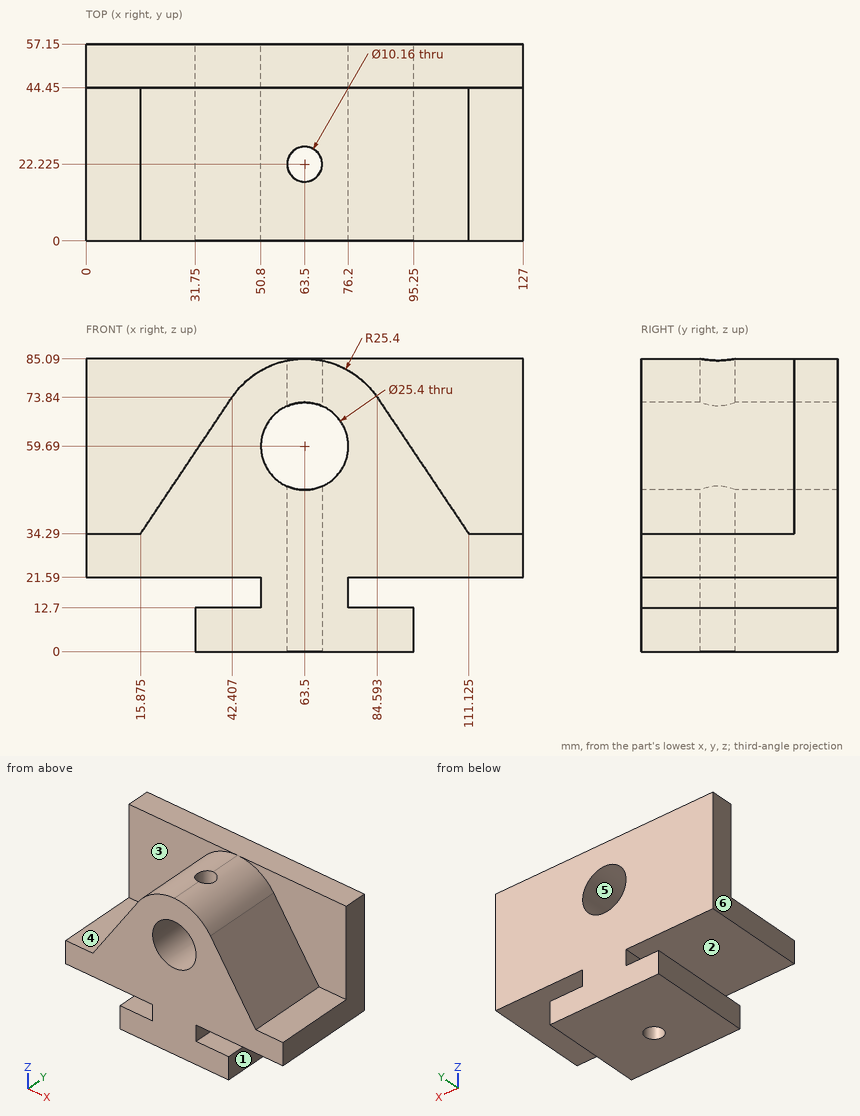
For this review, use the dimensioned drawing (mm, ordinates from the lowest corner) and the shaded views. A direction names the side the tool comes from. Give positions to 0.01 mm unless a question says otherwise; leave off trailing zeros. Use one line per item in the form item = value. Start each with the question number.
Item 1: To check wall thickness, follow line 1 along Z through (x, y) = (90.5, 46.5); line 2 along Z through (x, y) = (63.5, 12); line 3 along Y through (x, z) = (63, 76). State the ranges of each line that lie inside material, in increasing order. Write a range as from..to.
Item 2: For the marked faces 1, 2 and 3, list the 3-axis set-ups (+Z, -Z, +X, -X, +Y, -Y) from which the entire face can be reached by the end or side of a thin tool; tool diameter is ignored.
Item 3: Insertion check: pin 1 Ø1.5 at (x, y) = (36, 19.5) entering from +Z; pin 2 Ø5 at (x, y) = (25, 33) entering from +Z; pin 3 Ø15 at (x, y) = (86, 24) entering from +Z. Each pin has a flat end and moves straight along its axis. Give the tip position at first contact, or say it passes through.
Item 4: The part is to be moulded in two halves that separate along X. For the marked faces 4, 5 and 6, say which applies: pulls with the +X half, pulls with the -X half, needs draft (parallel to the pull), parting line crosses it, or undercut.
Completed:
q1.line_1 = 0..12.7, 21.59..85.09
q1.line_2 = 0..46.99, 72.39..85.09
q1.line_3 = 0..17.17, 27.28..57.15
q2.face_1 = -Z, +X, +Y, -Y
q2.face_2 = -X, +Y, -Y
q2.face_3 = +Z, -X, -Y
q3.pin_1 = 65.41
q3.pin_2 = 51.62
q3.pin_3 = 80.19
q4.face_4 = needs draft
q4.face_5 = undercut
q4.face_6 = pulls with the -X half
